Autodesk Inventor part; units mm, degrees
ref_plane "Work Plane1" through (29, 0, 0) normal (0, -1, 0) x (1, 0, 0)
ref_plane "YZ Plane" through (0, 0, 0) normal (1, 0, 0) x (0, 1, 0)
ref_plane "XZ Plane" through (0, 0, 0) normal (0, 1, 0) x (-1, 0, 0)
sketch "Sketch1" plane through (0, 0, 0) normal (0, 0, 1) x (1, 0, 0)
  line L0 (-0.5833, 0) -> (4, 0)
  line L1 (4, 0) -> (4, 1.25)
  line L2 (4, 1.25) -> (1.1761, 1.25)
  line L3 (1.1761, 1.25) -> (0.8999, 1.25)
  line L4 (0.8999, 1.25) -> (0, 1.25)
  line L5 (0, 1.25) -> (0, 2.25)
  line L6 (0, 2.25) -> (-2.5, 2.25)
  line L7 (-2.5, 2.25) -> (-2.5, 1.1547)
  line L8 (-2.5, 1.1547) -> (-1.25, 1.1547)
  line L9 (-1.25, 1.1547) -> (-0.5833, 0)
  line L10 (-3.8, 0) -> (5.3, 0)
  line L11 (0, -0.45) -> (0, 2.7)
  line L12 (1.1761, 1.25) -> (0, 1.25) construction
  dimension "d1" = 2.8239
  dimension "d2" = 0.2762
  dimension "d3" = 2.5
  dimension "d4" = 1.25
  dimension "d5" = 60
  dimension "d6" = 2.5
  dimension "d7" = 2.5
  dimension "d8" = 2.3094
  dimension "d9" = 4.5
  dimension "d26" = 4
revolve "Body" add sketch "Sketch1" angle 360 about axis through (-0.5833, 0, 0) along (1, 0, 0)
sketch "Sketch2" plane through (-2.5, 0, 0) normal (-1, 0, 0) x (0, 0, 1)
  circle A0 centre (0, 0) radius 1.1547
  line L0 (0, -3.15) -> (0, 3.15)
  line L1 (-3.15, 0) -> (3.15, 0)
  line L2 (1.1547, 0) -> (0.5774, -1)
  line L3 (0.5774, -1) -> (-0.5774, -1)
  line L4 (-0.5774, -1) -> (-1.1547, 0)
  line L5 (-1.1547, 0) -> (-0.5774, 1)
  line L6 (-0.5774, 1) -> (0.5774, 1)
  line L7 (0.5774, 1) -> (1.1547, 0)
extrude "Slot" add sketch "Sketch2" against normal up to next contours L7 A0 | A0 L2 | L6 L0 A0 | A0 L0 L3 | L0 L6 A0 | A0 L3 L0 | L4 A0 | A0 L5
fillet "Fillet1" radius 0.25 1 edges at (-2.5, -2.25, 0)
thread "Thread"
chamfer "Chamfer1" distance 0.2761 distance2 0.2761 1 edges at (4, -1.25, 0) measured on face at (4, -0.1825, -0.5629)
ref_plane "Work Plane1" through (29, 0, 0) normal (0, -1, 0) x (1, 0, 0)
fillet "Fillet2" radius 0.1 1 edges at (0, -1.25, 0)
equation "\"d30\" = R"
equation "\"d17\" = RR"
equation "\"d13\" = GEL"
equation "\"d15\" = -0.5 * SPD + 0.5 * GD"
equation "\"d16\" = GUL"
equation "\"d1\" = GEL"
equation "\"d3\" = KOH"
equation "\"d4\" = INTI"
equation "\"d6\" = GD"
equation "\"d7\" = BDM"
equation "\"d8\" = 1.1547 * SW"
equation "\"d9\" = KOD"
equation "\"d26\" = NLG"
equation "\"GD\" = NND"
equation "\"NLG\" = 4"
equation "\"GEL\" = 2.82395"
equation "\"KOD\" = 4.5"
equation "\"KOH\" = 2.5"
equation "\"INTI\" = 1.25"
equation "\"GAL\" = 0.61345 * PTC"
equation "\"GUL\" = 0.61345 * PTC"
equation "\"BDM\" = NND"
equation "\"SW\" = 2"
equation "\"RR\" = 0.25"
equation "\"SPD\" = 1.94789"
equation "\"R\" = 0.1"
equation "\"TOA\" = 30deg"
equation "\"THREADDIA\" = 2.5"
equation "\"PTC\" = 0.45"
equation "\"NND\" = 2.5"
equation "\"E0\" = 1.155 * SW"
equation "\"GD1\" = THREADDIA - 1.2269 * PTC"
properties part number "ANSI B18.3.1M - M2.5x0.45 x 4" material "Steel, Mild"
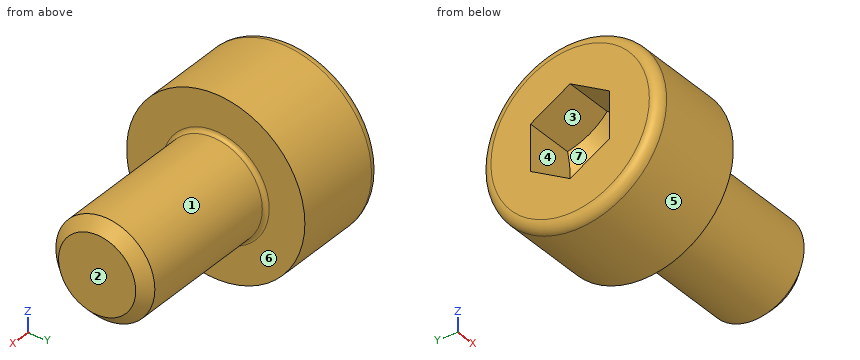
Input: part model. Units: mm. Frame: model coordinates. Face numbers are marked on the shaded views. A direction names the side the tool comes from. Give positions to 0.01 mm unless a question says otherwise; leave off trailing zeros. Order: outer loops, then holes, each group sorted by start corner. A loop starts at its lowest first (then second) coordinate and runs counter-clockwise, first axis right, second up. Notation, with made-up numbers: M -30.75,58.25 L 20.25,58.25 A18 ccw 20.25,82.25 Z; hole C 1,1.5 d4. An arc over 180 degrees is marked long. One line per question, with ' | ' between items. Start each with the question number.
1. Pull-direction query (Z, two-part tool) for the marked faces 4, 5, 6 and 7; classes: released by +Z, released by -Z, zero draft, split by the parting line, or undercut.
2. First-contact query: pin 1 Ø2 at (y, z) = (-1, 0) entering from +X; pin 2 Ø2 at (x, z) = (2.5, 0) entering from -Y; pin 3 Ø1 at (x, y) = (3.5, -1.5) entering from +Z. Flat tips, straight axial feed; report the tip coordinate or a pass-through.
3. Section query A-A (x = 1). Return the cut outline in (y, z).
4. Access query for the marked faces 1, 2 and 3. Directions: +Z, -Z, +X, -X, +Y, -Y. A direction counts if a zero-diameter tool reaches every point of the face in a straight line with its end or side. Return the directions, or none.
5. Material intervals for probe 1 along X at (y, z) = (1.4, -0.1); probe 2 along Z at (x, y) = (-2, 0.1); probe 3 along Y at (x, z) = (-1, -0.5), sorted ascending. Write a range as [from, to].
Here are the results:
1) face 4: undercut | face 5: split by the parting line | face 6: zero draft | face 7: undercut
2) pin 1: x = 4 | pin 2: y = -1.25 | pin 3: z = 0.75
3) outline: C 0,0 d2.5
4) face 1: +X | face 2: +Z, -Z, +X, +Y, -Y | face 3: -X
5) probe 1: [-2.5, 0] | probe 2: [-2.25, -1.1], [1.1, 2.25] | probe 3: [-2.19, -0.52], [0.52, 2.19]
